Verification items for this drawing (mm, ordinates from the low corner). A direction names the side the tool comes from. Round coordinates to 2 decimals unless told otherwise and drop trailing zeros. Order: outer loops, then holes, each group sorted by start corner. A loop starts at its lowest first (then second) coordinate and runs counter-clockwise, first axis right, second up. Notation, with made-up numbers: M 77,54.25 L 101,54.25 A12 cw 101,65.25 Z; hole C 43,-31 d1. An arc over 180 degrees is marked long. One line per item, written item: value. Start each with the question number.
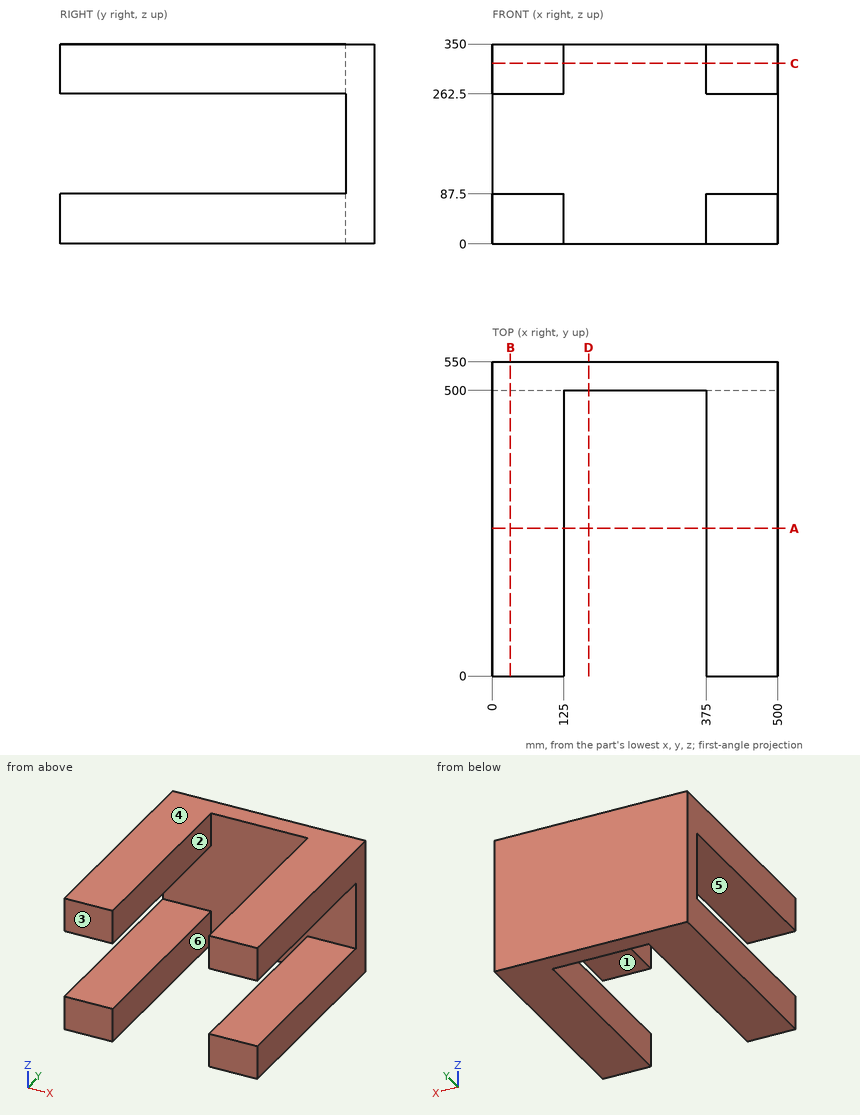
1. Depth check by flat-ended pin: pin 1 (3 mm diameter, centred on x = 308.5, z = 72, fed in from -Y). Enter the tip coordinate at first touch or a pass-through.
2. Tool access check on the marked faces 1, 2 and 3. Record the directions out of +Z, -Z, +X, -X, +Y, -Y that give a thin tool (end or side, any length) a straight path to the whole face; none if there is none.
3. Draft check along Z on the marked faces 4, 5 and 6. Enter one of: released by +Z, released by -Z, zero draft, split by the parting line, or undercut.
4. Section check A-A (y = 258.5). Record the cut outline in (x, z).
5. Section check B-B (x = 31.5). Record the cut outline in (y, z), and give its area (3 significant figures).
6. Scan lines: line 1 along Z through (x, y) = (106, 265.5); line 2 along X through (y, z) = (191, 314); line 3 along Y through (x, z) = (38, 142.5). Record each from-to range of solid material in increasing order.
7. Section check C-C (z = 316). Record the cut outline in (x, y).
8. Section check D-D (x = 168.5). Record the cut outline in (y, z), and give its area (3 significant figures).
Geometry check:
1. pin 1: stops at y = 500
2. face 1: +X, -X, -Y
2. face 2: +Z, -Z, -Y
2. face 3: +Z, -Z, +X, -X, -Y
3. face 4: released by +Z
3. face 5: undercut
3. face 6: zero draft
4. outline: M 0,0 L 125,0 L 125,87.5 L 0,87.5 Z; M 0,262.5 L 125,262.5 L 125,350 L 0,350 Z; M 375,0 L 500,0 L 500,87.5 L 375,87.5 Z; M 375,262.5 L 500,262.5 L 500,350 L 375,350 Z
5. outline: M 0,0 L 550,0 L 550,350 L 0,350 L 0,262.5 L 500,262.5 L 500,87.5 L 0,87.5 Z
5. area: 105,000 mm²
6. line 1: z = 0 to 87.5, 262.5 to 350
6. line 2: x = 0 to 125, 375 to 500
6. line 3: y = 500 to 550
7. outline: M 0,0 L 125,0 L 125,500 L 375,500 L 375,0 L 500,0 L 500,550 L 0,550 Z
8. outline: M 500,0 L 550,0 L 550,350 L 500,350 Z
8. area: 17,500 mm²
